Geometry check sheet. Reference: the model listing, model coordinates, mm. Face numbers are marked on the shaded views. A direction names the side the tool comes from. Give positions to 0.01 mm unless a question says otherwise; leave off trailing zeros. Order: outer loops, then holes, each group sorted by start corner. A loop starts at its lowest first (then second) coordinate and runs counter-clockwise, first axis right, second up. Notation, with made-up numbers: M 79.25,6 L 106.25,6 A26 cw 106.25,31 Z; hole C 12.5,2.5 d7. An arc over 180 degrees is marked long. Answer as CSV lines item,"result".
from build123d import *

# Parameters (mm, degrees)
BOX015_W     = 1
BOX015_H     = 1
BOX015_DEPTH = 1
BOX016_W     = 1
BOX016_H     = 1
BOX016_DEPTH = 1
BOX018_W     = 1
BOX018_H     = 1
BOX018_DEPTH = 1
BOX017_W     = 1
BOX017_H     = 1
BOX017_DEPTH = 1
BOX014_W     = 3
BOX014_H     = 3
BOX014_DEPTH = 7
BOX024_W     = 9
BOX024_H     = 1
BOX024_DEPTH = 4
BOX020_W     = 1
BOX020_H     = 1
BOX020_DEPTH = 1
BOX021_W     = 1
BOX021_H     = 1
BOX021_DEPTH = 1
BOX023_W     = 1
BOX023_H     = 1
BOX023_DEPTH = 1
BOX022_W     = 1
BOX022_H     = 1
BOX022_DEPTH = 1
BOX019_W     = 3
BOX019_H     = 3
BOX019_DEPTH = 7
BOX003_W     = 9
BOX003_H     = 1
BOX003_DEPTH = 4
BOX004_W     = 9
BOX004_H     = 1
BOX004_DEPTH = 4
BOX010_W     = 1
BOX010_H     = 1
BOX010_DEPTH = 1
BOX011_W     = 1
BOX011_H     = 1
BOX011_DEPTH = 1
BOX013_W     = 1
BOX013_H     = 1
BOX013_DEPTH = 1
BOX012_W     = 1
BOX012_H     = 1
BOX012_DEPTH = 1
BOX009_W     = 3
BOX009_H     = 3
BOX009_DEPTH = 7
BOX005_W     = 1
BOX005_H     = 1
BOX005_DEPTH = 1
BOX006_W     = 1
BOX006_H     = 1
BOX006_DEPTH = 1
BOX008_W     = 1
BOX008_H     = 1
BOX008_DEPTH = 1
BOX007_W     = 1
BOX007_H     = 1
BOX007_DEPTH = 1
BOX001_W     = 3
BOX001_H     = 3
BOX001_DEPTH = 7
BOX025_W     = 3
BOX025_H     = 1
BOX025_DEPTH = 3
BOX_W        = 9
BOX_H        = 1
BOX_DEPTH    = 4


with BuildPart() as cubo015:
    # Box015 → Box015 (new body)
    with BuildSketch(Plane(origin=(-1, 1, 7), x_dir=(1, 0, 0), z_dir=(0, 0, 1))):
        with Locations((0.5, 0.5)):
            Rectangle(BOX015_W, BOX015_H)
    extrude(amount=BOX015_DEPTH)


with BuildPart() as cubo016:
    # Box016 → Box016 (new body)
    with BuildSketch(Plane(origin=(-1, -1, 7), x_dir=(1, 0, 0), z_dir=(0, 0, 1))):
        with Locations((0.5, 0.5)):
            Rectangle(BOX016_W, BOX016_H)
    extrude(amount=BOX016_DEPTH)


with BuildPart() as cubo018:
    # Box018 → Box018 (new body)
    with BuildSketch(Plane(origin=(-3, 1, 7), x_dir=(1, 0, 0), z_dir=(0, 0, 1))):
        with Locations((0.5, 0.5)):
            Rectangle(BOX018_W, BOX018_H)
    extrude(amount=BOX018_DEPTH)


with BuildPart() as cubo017:
    # Box017 → Box017 (new body)
    with BuildSketch(Plane(origin=(-3, -1, 7), x_dir=(1, 0, 0), z_dir=(0, 0, 1))):
        with Locations((0.5, 0.5)):
            Rectangle(BOX017_W, BOX017_H)
    extrude(amount=BOX017_DEPTH)


with BuildPart() as fusion011:
    # Box014 → Box014 (new body)
    with BuildSketch(Plane(origin=(-3, -1, 0), x_dir=(1, 0, 0), z_dir=(0, 0, 1))):
        with Locations((1.5, 1.5)):
            Rectangle(BOX014_W, BOX014_H)
    extrude(amount=BOX014_DEPTH)

    # Fusion008: union Cubo017
    add(cubo017.part)

    # Fusion009: union Cubo018
    add(cubo018.part)

    # Fusion010: union Cubo016
    add(cubo016.part)

    # Fusion011: union Cubo015
    add(cubo015.part)


with BuildPart() as fusion011_1:
    # Fusion011 placement: moved
    add(fusion011.part.moved(Location((12, 12, 0))))


with BuildPart() as cubo024:
    # Box024 → Box024 (new body)
    with BuildSketch(Plane(origin=(0, 12, 0), x_dir=(1, 0, 0), z_dir=(0, 0, 1))):
        with Locations((4.5, 0.5)):
            Rectangle(BOX024_W, BOX024_H)
    extrude(amount=BOX024_DEPTH)


with BuildPart() as cubo020:
    # Box020 → Box020 (new body)
    with BuildSketch(Plane(origin=(-1, 1, 7), x_dir=(1, 0, 0), z_dir=(0, 0, 1))):
        with Locations((0.5, 0.5)):
            Rectangle(BOX020_W, BOX020_H)
    extrude(amount=BOX020_DEPTH)


with BuildPart() as cubo021:
    # Box021 → Box021 (new body)
    with BuildSketch(Plane(origin=(-1, -1, 7), x_dir=(1, 0, 0), z_dir=(0, 0, 1))):
        with Locations((0.5, 0.5)):
            Rectangle(BOX021_W, BOX021_H)
    extrude(amount=BOX021_DEPTH)


with BuildPart() as cubo023:
    # Box023 → Box023 (new body)
    with BuildSketch(Plane(origin=(-3, 1, 7), x_dir=(1, 0, 0), z_dir=(0, 0, 1))):
        with Locations((0.5, 0.5)):
            Rectangle(BOX023_W, BOX023_H)
    extrude(amount=BOX023_DEPTH)


with BuildPart() as cubo022:
    # Box022 → Box022 (new body)
    with BuildSketch(Plane(origin=(-3, -1, 7), x_dir=(1, 0, 0), z_dir=(0, 0, 1))):
        with Locations((0.5, 0.5)):
            Rectangle(BOX022_W, BOX022_H)
    extrude(amount=BOX022_DEPTH)


with BuildPart() as fusion015:
    # Box019 → Box019 (new body)
    with BuildSketch(Plane(origin=(-3, -1, 0), x_dir=(1, 0, 0), z_dir=(0, 0, 1))):
        with Locations((1.5, 1.5)):
            Rectangle(BOX019_W, BOX019_H)
    extrude(amount=BOX019_DEPTH)

    # Fusion012: union Cubo022
    add(cubo022.part)

    # Fusion013: union Cubo023
    add(cubo023.part)

    # Fusion014: union Cubo021
    add(cubo021.part)

    # Fusion015: union Cubo020
    add(cubo020.part)


with BuildPart() as fusion015_1:
    # Fusion015 placement: moved
    add(fusion015.part.moved(Location((0, 12, 0))))


with BuildPart() as cubo003:
    # Box003 → Box003 (new body)
    with BuildSketch(Plane(origin=(-1, 2, 0), x_dir=(0, 1, 0), z_dir=(0, 0, 1))):
        with Locations((4.5, 0.5)):
            Rectangle(BOX003_W, BOX003_H)
    extrude(amount=BOX003_DEPTH)


with BuildPart() as cubo004:
    # Box004 → Box004 (new body)
    with BuildSketch(Plane(origin=(11, 2, 0), x_dir=(0, 1, 0), z_dir=(0, 0, 1))):
        with Locations((4.5, 0.5)):
            Rectangle(BOX004_W, BOX004_H)
    extrude(amount=BOX004_DEPTH)


with BuildPart() as cubo010:
    # Box010 → Box010 (new body)
    with BuildSketch(Plane(origin=(-1, 1, 7), x_dir=(1, 0, 0), z_dir=(0, 0, 1))):
        with Locations((0.5, 0.5)):
            Rectangle(BOX010_W, BOX010_H)
    extrude(amount=BOX010_DEPTH)


with BuildPart() as cubo011:
    # Box011 → Box011 (new body)
    with BuildSketch(Plane(origin=(-1, -1, 7), x_dir=(1, 0, 0), z_dir=(0, 0, 1))):
        with Locations((0.5, 0.5)):
            Rectangle(BOX011_W, BOX011_H)
    extrude(amount=BOX011_DEPTH)


with BuildPart() as cubo013:
    # Box013 → Box013 (new body)
    with BuildSketch(Plane(origin=(-3, 1, 7), x_dir=(1, 0, 0), z_dir=(0, 0, 1))):
        with Locations((0.5, 0.5)):
            Rectangle(BOX013_W, BOX013_H)
    extrude(amount=BOX013_DEPTH)


with BuildPart() as cubo012:
    # Box012 → Box012 (new body)
    with BuildSketch(Plane(origin=(-3, -1, 7), x_dir=(1, 0, 0), z_dir=(0, 0, 1))):
        with Locations((0.5, 0.5)):
            Rectangle(BOX012_W, BOX012_H)
    extrude(amount=BOX012_DEPTH)


with BuildPart() as fusion007:
    # Box009 → Box009 (new body)
    with BuildSketch(Plane(origin=(-3, -1, 0), x_dir=(1, 0, 0), z_dir=(0, 0, 1))):
        with Locations((1.5, 1.5)):
            Rectangle(BOX009_W, BOX009_H)
    extrude(amount=BOX009_DEPTH)

    # Fusion004: union Cubo012
    add(cubo012.part)

    # Fusion005: union Cubo013
    add(cubo013.part)

    # Fusion006: union Cubo011
    add(cubo011.part)

    # Fusion007: union Cubo010
    add(cubo010.part)


with BuildPart() as fusion007_1:
    # Fusion007 placement: moved
    add(fusion007.part.moved(Location((12, 0, 0))))


with BuildPart() as cubo005:
    # Box005 → Box005 (new body)
    with BuildSketch(Plane(origin=(-1, 1, 7), x_dir=(1, 0, 0), z_dir=(0, 0, 1))):
        with Locations((0.5, 0.5)):
            Rectangle(BOX005_W, BOX005_H)
    extrude(amount=BOX005_DEPTH)


with BuildPart() as cubo006:
    # Box006 → Box006 (new body)
    with BuildSketch(Plane(origin=(-1, -1, 7), x_dir=(1, 0, 0), z_dir=(0, 0, 1))):
        with Locations((0.5, 0.5)):
            Rectangle(BOX006_W, BOX006_H)
    extrude(amount=BOX006_DEPTH)


with BuildPart() as cubo008:
    # Box008 → Box008 (new body)
    with BuildSketch(Plane(origin=(-3, 1, 7), x_dir=(1, 0, 0), z_dir=(0, 0, 1))):
        with Locations((0.5, 0.5)):
            Rectangle(BOX008_W, BOX008_H)
    extrude(amount=BOX008_DEPTH)


with BuildPart() as cubo007:
    # Box007 → Box007 (new body)
    with BuildSketch(Plane(origin=(-3, -1, 7), x_dir=(1, 0, 0), z_dir=(0, 0, 1))):
        with Locations((0.5, 0.5)):
            Rectangle(BOX007_W, BOX007_H)
    extrude(amount=BOX007_DEPTH)


with BuildPart() as fusion003:
    # Box001 → Box001 (new body)
    with BuildSketch(Plane(origin=(-3, -1, 0), x_dir=(1, 0, 0), z_dir=(0, 0, 1))):
        with Locations((1.5, 1.5)):
            Rectangle(BOX001_W, BOX001_H)
    extrude(amount=BOX001_DEPTH)

    # Fusion: union Cubo007
    add(cubo007.part)

    # Fusion001: union Cubo008
    add(cubo008.part)

    # Fusion002: union Cubo006
    add(cubo006.part)

    # Fusion003: union Cubo005
    add(cubo005.part)


with BuildPart() as cubo025:
    # Box025 → Box025 (new body)
    with BuildSketch(Plane(origin=(3, 0, 0), x_dir=(1, 0, 0), z_dir=(0, 0, 1))):
        with Locations((1.5, 0.5)):
            Rectangle(BOX025_W, BOX025_H)
    extrude(amount=BOX025_DEPTH)


with BuildPart() as fusion022:
    # Box → Box (new body)
    with BuildSketch(Plane.XY):
        with Locations((4.5, 0.5)):
            Rectangle(BOX_W, BOX_H)
    extrude(amount=BOX_DEPTH)

    # Cut: cut Cubo025
    add(cubo025.part, mode=Mode.SUBTRACT)

    # Fusion016: union Fusion003
    add(fusion003.part)

    # Fusion017: union Fusion007
    add(fusion007_1.part)

    # Fusion018: union Cubo004
    add(cubo004.part)

    # Fusion019: union Cubo003
    add(cubo003.part)

    # Fusion020: union Fusion015
    add(fusion015_1.part)

    # Fusion021: union Cubo024
    add(cubo024.part)

    # Fusion022: union Fusion011
    add(fusion011_1.part)


solid = fusion022.part
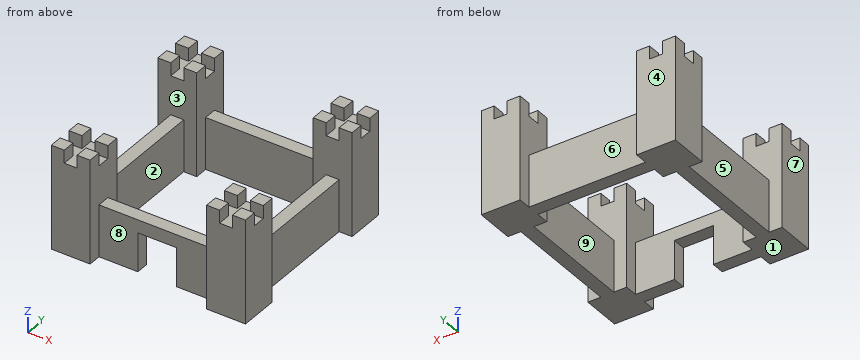
(1) Section check B-B on y = 5.25. Enter the section's corners in (x, z).
The answers:
outline,"M -2,0 L -1,0 L -1,4 L -2,4 Z; M 10,0 L 11,0 L 11,4 L 10,4 Z"
(2) Gauge pin test, flat ends, axial feed: P1, Ø3, axis at x = 7, z = 2, coming from the -Y side; P2, Ø4, axis at y = 8, z = 3.5, coming from the +X side; P3, Ø4.5, axis at y = 4.5, z = 2.5, coming from the -X side; P4, Ø3.5, axis at x = 10.5, y = 13, coming from the +Z side. Record the tip position at first contact, or that the pin passes through.
The answers:
P1,"stops at y = 0"
P2,"stops at x = 11"
P3,"stops at x = -2"
P4,"stops at z = 8"
(3) Section check D-D on y = 11.5. Enter the section's corners in (x, z).
The answers:
outline,"M -3,0 L 0,0 L 0,8 L -1,8 L -1,7 L -2,7 L -2,8 L -3,8 Z; M 9,0 L 12,0 L 12,8 L 11,8 L 11,7 L 10,7 L 10,8 L 9,8 Z"
(4) Draft check along Y on the marked faces 6, 7, 8 and 9. Enter one of: +Y half, -Y half, draft (parallel to the pull), parting line (faces both ways), or undercut.
The answers:
face 6,"+Y half"
face 7,"draft"
face 8,"-Y half"
face 9,"undercut"
(5) Section check A-A on x = 11.25. Enter the section's corners in (y, z).
The answers:
outline,"M -1,0 L 2,0 L 2,8 L 1,8 L 1,7 L 0,7 L 0,8 L -1,8 Z; M 11,0 L 14,0 L 14,8 L 13,8 L 13,7 L 12,7 L 12,8 L 11,8 Z"
(6) Tool access check on the marked faces 1, 2, 3, 4 and 5. Record the directions out of +Z, -Z, +X, -X, +Y, -Y that give a thin tool (end or side, any length) a straight path to the whole face; none if there is none.
The answers:
face 1,"-Z, +X, -X, +Y, -Y"
face 2,"+Z, -Z"
face 3,"+Z"
face 4,"+Z, -Z, +X, -X, +Y"
face 5,"+Z, -Z, -X"
(7) Section check C-C on x = 1.75. Enter the section's corners in (y, z), then the cut area to 3 significant figures.
The answers:
outline,"M 0,0 L 1,0 L 1,4 L 0,4 Z; M 12,0 L 13,0 L 13,4 L 12,4 Z"
area,"8.00 mm2"
(8) Material ranges on line 1 (Y direction, x = 9.5, z = 2.5); line 2 (X direction, y = 13.25, z = 5); line 3 (X direction, y = 8.75, z = 1.75), recorded low to high.
The answers:
line 1,"y = -1 to 2, 11 to 14"
line 2,"x = -3 to 0, 9 to 12"
line 3,"x = -2 to -1, 10 to 11"
